Source: CAD feature listing. Evaluate the final solid. Frame: model axes, mm. Face numbers are marked on the shaded views. A direction names the side the tool comes from. Give positions to 0.01 mm unless a question says otherwise; leave off trailing zeros. Write each loop counter-clockwise with the first axis right and the second up, starting at its lowest first coordinate (ties: lowest second). Pieces come first, ordered by that corner, then holes. Notation, with made-up numbers: (-31, -27) - (11, -27) arc R15 ccw to (11, -1) - close; hole circle Ø7 at (34, -38). An arc over 180 degrees is marked (long way). Answer as a JSON object with one key per item and string values. Group by question number.
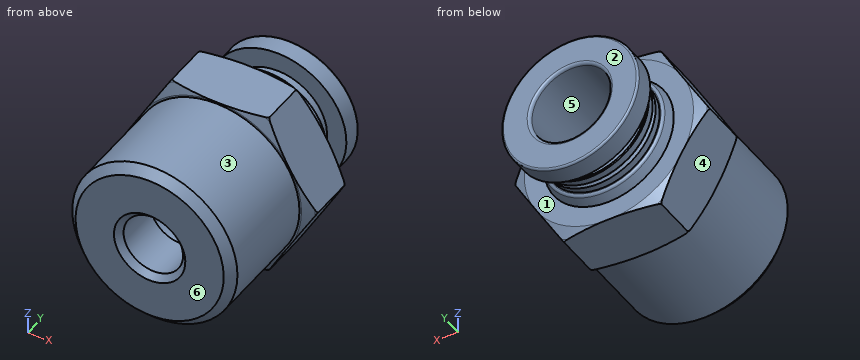
from build123d import *

# Parameters (mm, degrees)
SKETCH_2_R          = 11.814954576
CUT_EXTRUDE_1_DEPTH = 23


with BuildPart() as part:
    # 草图1 → 旋转1 (revolve)
    with BuildSketch(Plane.XY, mode=Mode.PRIVATE) as revolve_1_sk:
        with BuildLine():
            Line((3, 5), (3, 0.6))
            Line((3, 0.6), (3.6, 0))
            Line((3.6, 0), (7.475, 0))
            Line((7.475, 0), (8.331, 0.856))
            Line((8.331, 0.856), (8.331, 11))
            Line((8.331, 11), (8.534954576, 11))
            Line((8.534954576, 11), (9.629759606, 11.453483091))
            ThreePointArc((9.629759606, 11.453483091), (9.76439546, 11.563975881), (9.814954576, 11.730646951))
            Line((9.814954576, 11.730646951), (9.814954576, 15.869353049))
            ThreePointArc((9.814954576, 15.869353049), (9.76439546, 16.036024119), (9.629759606, 16.146516909))
            Line((9.629759606, 16.146516909), (8.534954576, 16.6))
            Line((8.534954576, 16.6), (6.55, 16.6))
            Line((6.55, 16.6), (6.215570396, 17.504080695))
            ThreePointArc((6.215570396, 17.504080695), (6.105632697, 17.646195256), (5.934203715, 17.7))
            Line((5.934203715, 17.7), (5.8, 17.7))
            Line((5.8, 17.7), (5.8, 18.36))
            Line((5.8, 18.36), (5.56, 18.6))
            Line((5.56, 18.6), (5.8, 18.84))
            Line((5.8, 18.84), (5.8, 19.5))
            Line((5.8, 19.5), (5.7, 19.6))
            Line((5.7, 19.6), (4.95, 19.6))
            Line((4.95, 19.6), (4.95, 21))
            Line((4.95, 21), (6.9, 21))
            Line((6.9, 21), (6.9, 22.8))
            ThreePointArc((6.9, 22.8), (6.841421356, 22.941421356), (6.7, 23))
            Line((6.7, 23), (4.3, 23))
            ThreePointArc((4.3, 23), (4.087867966, 22.912132034), (4, 22.7))
            Line((4, 22.7), (4, 5))
            Line((4, 5), (3, 5))
        make_face()
    revolve(revolve_1_sk.sketch.rotate(Axis((0, 0, 0), (0, 1, 0)), 270), axis=Axis((0, 0, 0), (0, 1, 0)))

    # 草图2 → 切除-拉伸1 (cut)
    with BuildSketch(Plane(origin=(0, 11, 0), x_dir=(1, 0, 0), z_dir=(0, 1, 0))):
        Circle(SKETCH_2_R)
        Polygon((-9.814954576, 0), (-4.907477288, -8.5), (4.907477288, -8.5), (9.814954576, 0), (4.907477288, 8.5), (-4.907477288, 8.5), align=None, mode=Mode.SUBTRACT)
    extrude(amount=CUT_EXTRUDE_1_DEPTH, mode=Mode.SUBTRACT)


solid = part.part
Q1. Reachability of the marked faces 1, 2 and 3 from +Z, -Z, +X, -X, +Y, -Y: full face, straight path, thin tool, end or side. Return the list, or none.
Q2. Section C-C on y = 3. Return the cut outline in (x, z), then the cut area to 3 significant figures.
Q3. Section B-B on y = 7.25. Return the cut outline in (x, z), then the cut area to 3 significant figures.
Q4. Ray query, probe 1 along X at (y, z) = (1.75, 0); probe 2 along Y at (x, z) = (3, 4.5); probe 3 along Y at (x, z) = (5.5, -2.25). Return the intervals inside material, ascending. Write a range as [from, to].
Q5. Draft query along X for the marked faces 4, 5 and 6. Return one class per face: released by +X, released by -X, zero draft, split by the parting line, or undercut.
Q6. First-contact query: pin 1 Ø10 at (y, z) = (4, 5.5) entering from +X; pin 2 Ø1.5 at (x, z) = (0, -1) entering from -Y; pin 3 Ø1.5 at (y, z) = (16, 2) entering from +X; pin 4 Ø4 at (x, z) = (3, -3) entering from -Y. Flat tips, straight axial feed; report the tip coordinate or a pass-through.
Q7. Section A-A on y = 14.25. Return the cut outline in (x, z), then the cut area to 3 significant figures.
Taken from the geometry:
{
 "1": {"face 1": "none", "face 2": "+Z, -Z, +X, -X, +Y", "face 3": "-Y"},
 "2": {"outline": "circle Ø16.66 at (0, 0); hole circle Ø6 at (0, 0)", "area": "190 mm²"},
 "3": {"outline": "circle Ø16.66 at (0, 0); hole circle Ø8 at (0, 0)", "area": "168 mm²"},
 "4": {"probe 1": "x = [-8.33, -3], [3, 8.33]", "probe 2": "y = [0, 19.6], [21, 23]", "probe 3": "y = [0, 17.7], [21, 23]"},
 "5": {"face 4": "released by -X", "face 5": "undercut", "face 6": "zero draft"},
 "6": {"pin 1": "stops at x = 8.32", "pin 2": "passes through", "pin 3": "stops at x = 9.09", "pin 4": "stops at y = 0"},
 "7": {"outline": "(-9.81, 0) - (-4.91, -8.5) - (4.91, -8.5) - (9.81, 0) - (4.91, 8.5) - (-4.91, 8.5) - close; hole circle Ø8 at (0, 0)", "area": "200 mm²"}
}
